```python
from build123d import *

# Parameters (mm, degrees)
EXTRUDE_1_DEPTH     = 12
SKETCH_2_R          = 10.5
SKETCH_2_R_2        = 34.6
SKETCH_2_R_3        = 2.1
CUT_EXTRUDE_1_DEPTH = 12
FILLET_1_R          = 10
SKETCH_3_W          = 22
SKETCH_3_H          = 50
CUT_EXTRUDE_2_DEPTH = 12
FILLET_2_R          = 10
CUT_EXTRUDE_3_DEPTH = 264.96969523
FILLET_4_R          = 4


with BuildPart() as part:
    # 草图1 → 凸台-拉伸1 (new body)
    with BuildSketch(Plane.XY):
        with BuildLine():
            Line((-17.5, 40.370162249), (-19.998429914, 239.749398802))
            ThreePointArc((-19.998429914, 239.749398802), (0, 260), (19.998429914, 239.749398802))
            Line((19.998429914, 239.749398802), (17.5, 40.370162249))
            ThreePointArc((17.5, 40.370162249), (0, -44), (-17.5, 40.370162249))
        make_face()
    extrude(amount=EXTRUDE_1_DEPTH)

    # 草图2 → 切除-拉伸1 (cut)
    with BuildSketch(Plane.XY.offset(12)):
        with Locations((0, 240)):
            Circle(SKETCH_2_R)
        Circle(SKETCH_2_R_2)
        with Locations((20, 34.641016151)):
            Circle(SKETCH_2_R_3)
        with Locations((40, 0)):
            Circle(SKETCH_2_R_3)
        with Locations((20, -34.641016151)):
            Circle(SKETCH_2_R_3)
        with Locations((-20, -34.641016151)):
            Circle(SKETCH_2_R_3)
        with Locations((-40, 0)):
            Circle(SKETCH_2_R_3)
        with Locations((-20, 34.641016151)):
            Circle(SKETCH_2_R_3)
    extrude(amount=-CUT_EXTRUDE_1_DEPTH, mode=Mode.SUBTRACT)

    # 圆角1
    fillet_1_edges = [part.edges().sort_by_distance(p)[0] for p in [
        (-17.5, 40.370162249, 6),
        (17.5, 40.370162249, 6),
    ]]
    fillet(fillet_1_edges, radius=FILLET_1_R)

    # 草图3 → 切除-拉伸2 (cut)
    with BuildSketch(Plane(origin=(0, 0, 0), x_dir=(-1, 0, 0), z_dir=(0, 0, -1))):
        with Locations((0, 50)):
            Rectangle(SKETCH_3_W, SKETCH_3_H)
    extrude(amount=-CUT_EXTRUDE_2_DEPTH, mode=Mode.SUBTRACT)

    # 圆角2
    fillet_2_edges = [part.edges().sort_by_distance(p)[0] for p in [
        (-11, 32.804877686, 6),
        (11, 32.804877686, 6),
        (-11, 75, 6),
        (11, 75, 6),
    ]]
    fillet(fillet_2_edges, radius=FILLET_2_R)

    # 草图5 → 切除-拉伸3 (cut, through all)
    with BuildSketch(Plane(origin=(0, 0, 0), x_dir=(-1, 0, 0), z_dir=(0, 0, -1))):
        Polygon((-13.775012743, 221.957895182), (16.705979035, 204.93348865), (-12.897497215, 151.930565202), align=None)
        Polygon((13.279210594, 182.391984789), (-10.08410037, 140.561634461), (12.649095231, 132.107636495), align=None)
        Polygon((-12.660080973, 132.98431864), (11.431866329, 124.025029456), (-12.071548884, 86.018390981), align=None)
    extrude(amount=-CUT_EXTRUDE_3_DEPTH, mode=Mode.SUBTRACT)

    # 圆角4
    fillet_4_edges = [part.edges().sort_by_distance(p)[0] for p in [
        (-13.279210594, 182.391984789, 6),
        (-12.649095231, 132.107636495, 6),
        (10.08410037, 140.561634461, 6),
        (12.071548884, 86.018390981, 6),
        (12.660080973, 132.98431864, 6),
        (-11.431866329, 124.025029456, 6),
        (12.897497215, 151.930565202, 6),
        (13.775012743, 221.957895182, 6),
        (-16.705979035, 204.93348865, 6),
    ]]
    fillet(fillet_4_edges, radius=FILLET_4_R)


solid = part.part
```
Part model, mm, in its own coordinate system. A direction names the side the tool comes from. Coordinates: 2 decimals unless noted, no trailing zeros. Order: outer loops, then holes, each group sorted by start corner. A loop starts at its lowest first (then second) coordinate and runs counter-clockwise, first axis right, second up. Notation, with made-up numbers: (-25, 85.5) -> (26, 85.5) arc R23 cw to (26, 105.5) -> close; hole circle Ø11 at (44.5, -34.75). An arc over 180 degrees is marked (long way). Put each result on its own line as item: value. Start each with the question number.
(1) Probe line 1 along Y through (x, z) = (0, 6); line 2 along Y through (x, z) = (5, 2.25); line 3 along X through (y, z) = (63, 7). List the from-to ranges inside material, lowest first. Write a range as [from, to].
(2) Band-saw the part on B-B (z = 5). Count the separate pieces of the cut face and the enclosed holes in it, then the cut area to 3 significant figures.
(3) Band-saw the part on C-C (y = 80). Give the cut face in (x, z), then the cut area to 3 significant figures.
(4) Which spindle directions (+Z, -Z, +X, -X, +Y, -Y) get a long thin tool onto all of the face, cutting with end or side? Do faces 3 (the face through (-4.724, 183.48, 5.916)), 4 (the face through (-18.82, 41.6, 6.08)). Say none if no direction does.
(5) Band-saw the part on A-A (y = 11.5). Give the cut face in (x, z).
(6) Mould opens along Y. For faces 1 (the face through (-3, 109, 12)), 2 (the face through (-15.124, 204.44, 6.084)) say: pulls with the +Y half, pulls with the -Y half, needs draft (parallel to the pull), parting line crosses it, or undercut.
(7) Pin check, flat tips, straight feed: pin 1 Ø5 at (x, z) = (25, 10) entering from -Y; pin 2 Ø5 at (x, z) = (33, 7) entering from +Y; pin 3 Ø1.5 at (y, z) = (197.5, 8.5) entering from -X; pin 4 Ø6.5 at (x, y) = (20, -34.64) entering from -Z. Stop position of each tip, or through.
Determined:
1. line 1: y = [-44, -34.6], [75, 105.54], [128.28, 136.81], [158.62, 175.02], [214.26, 229.5], [250.5, 260]
1. line 2: y = [-43.71, -34.24], [74.17, 97.47], [130.14, 138.67], [149.66, 166.07], [217.06, 230.77], [249.23, 259.36]
1. line 3: x = [-17.78, -11], [11, 17.78]
2. separate pieces: 1
2. enclosed holes: 11
2. area: 7,020 mm²
3. outline: (-18, 0) -> (18, 0) -> (18, 12) -> (-18, 12) -> close
3. area: 432 mm²
4. face 3: +Z, -Z
4. face 4: +Z, -Z, -X
5. outline: (-42.47, 0) -> (-32.63, 0) -> (-32.63, 12) -> (-42.47, 12) -> close; (32.63, 0) -> (42.47, 0) -> (42.47, 12) -> (32.63, 12) -> close
6. face 1: needs draft
6. face 2: undercut
7. pin 1: stops at y = -37.81
7. pin 2: stops at y = 31.71
7. pin 3: stops at x = -19.48
7. pin 4: stops at z = 0
